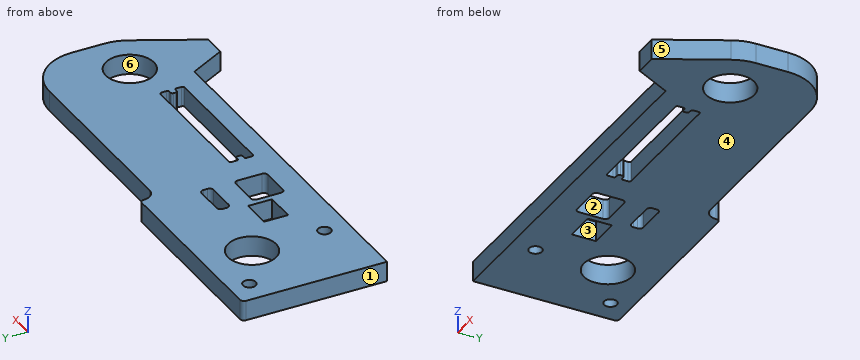
```python
from build123d import *

# Parameters (mm, degrees)
SKETCH1_R           = 5.98
SKETCH1_R_2         = 1.6
SKETCH1_W           = 9
SKETCH1_H           = 8
SKETCH1_H_2         = 3
SKETCH1_W_2         = 7.5
SKETCH1_H_3         = 6
BOSS_EXTRUDE1_DEPTH = 5
FILLET1_R           = 1
FILLET2_R           = 3
FILLET3_R           = 1
CUT_EXTRUDE1_DEPTH  = 98.867257037
FILLET4_R           = 0.5


with BuildPart() as part:
    # Sketch1 → Boss-Extrude1 (new body)
    with BuildSketch(Plane.XY):
        with BuildLine():
            Line((72.356568311, -24), (77.172081726, -33))
            Line((77.172081726, -33), (82.827918274, -33))
            Line((82.827918274, -33), (90.70873293, -17.415075165))
            ThreePointArc((90.70873293, -17.415075165), (91.67272023, -14.78345153), (92, -12))
            Line((92, -12), (92, -4))
            ThreePointArc((92, -4), (88.485281374, 4.485281374), (80, 8))
            Line((80, 8), (30, 8))
            Line((30, 8), (30, 12))
            Line((30, 12), (-18, 12))
            Line((-18, 12), (-18, -24))
            Line((-18, -24), (72.356568311, -24))
        make_face()
        Circle(SKETCH1_R, mode=Mode.SUBTRACT)
        with Locations((80, -12)):
            Circle(SKETCH1_R, mode=Mode.SUBTRACT)
        with Locations((-12, 7)):
            Circle(SKETCH1_R_2, mode=Mode.SUBTRACT)
        with Locations((0, -18)):
            Circle(SKETCH1_R_2, mode=Mode.SUBTRACT)
        with Locations((23, -14)):
            Rectangle(SKETCH1_W, SKETCH1_H, mode=Mode.SUBTRACT)
        with Locations((23, -3)):
            Rectangle(SKETCH1_W, SKETCH1_H_2, mode=Mode.SUBTRACT)
        with Locations((13.25, -11)):
            Rectangle(SKETCH1_W_2, SKETCH1_H_3, mode=Mode.SUBTRACT)
    extrude(amount=BOSS_EXTRUDE1_DEPTH)

    # Fillet1
    fillet1_edges = [part.edges().sort_by_distance(p)[0] for p in [
        (18.5, -10, 2.5),
        (18.5, -18, 2.5),
        (27.5, -18, 2.5),
        (27.5, -10, 2.5),
        (18.5, -1.5, 2.5),
        (18.5, -4.5, 2.5),
        (27.5, -4.5, 2.5),
        (27.5, -1.5, 2.5),
    ]]
    fillet(fillet1_edges, radius=FILLET1_R)

    # Fillet2
    fillet2_edges = [part.edges().sort_by_distance(p)[0] for p in [
        (30, 8, 2.5),
    ]]
    fillet(fillet2_edges, radius=FILLET2_R)

    # Fillet3
    fillet3_edges = [part.edges().sort_by_distance(p)[0] for p in [
        (30, 12, 2.5),
        (-18, 12, 2.5),
    ]]
    fillet(fillet3_edges, radius=FILLET3_R - 0.0001)  # a hair under: the kernel refuses the full size

    # Sketch2 → Cut-Extrude1 (cut, through all)
    with BuildSketch(Plane.XY.offset(5)):
        Polygon((35, -13), (68, -13), (68, -15.25), (66.5, -15.25), (66.5, -16.75), (68, -16.75), (68, -19), (35, -19), (35, -16.75), (36.5, -16.75), (36.5, -15.25), (35, -15.25), align=None)
    extrude(amount=-CUT_EXTRUDE1_DEPTH, mode=Mode.SUBTRACT)

    # Fillet4
    fillet4_edges = [part.edges().sort_by_distance(p)[0] for p in [
        (35, -15.25, 2.5),
        (35, -13, 2.5),
        (68, -13, 2.5),
        (68, -15.25, 2.5),
        (66.5, -15.25, 2.5),
        (66.5, -16.75, 2.5),
        (68, -16.75, 2.5),
        (68, -19, 2.5),
        (35, -19, 2.5),
        (35, -16.75, 2.5),
        (36.5, -16.75, 2.5),
        (36.5, -15.25, 2.5),
    ]]
    fillet(fillet4_edges, radius=FILLET4_R)


solid = part.part
```
Input: part model. Units: mm. Frame: model coordinates. Face numbers are marked on the shaded views. A direction names the side the tool comes from. Coordinates: 2 decimals unless noted, no trailing zeros. Loops run counter-clockwise (first coordinate to the right, second up) from the corner with the lowest first, then second, coordinate; pieces in that order, holes last. Notation, with made-up numbers: M 11,60.5 L 23,60.5 A31 cw 23,84.5 Z; hole C 52,-32 d10. An arc over 180 degrees is marked long. Answer in a Markdown table with one row per item.
1. Section A-A, the plane x = 46. Output: boundary loops of the cut face in (y, z).
Response:
| item | result |
|---|---|
| outline | M -24,0 L -19,0 L -19,5 L -24,5 Z; M -13,0 L 8,0 L 8,5 L -13,5 Z |
2. First-contact query: pin 1 (2 mm diameter, centred on x = 27, y = 3, fed in from -Z); pin 2 (11 mm diameter, centred on x = 0, y = 0, fed in from +Z); pin 3 (1 mm diameter, centred on x = 32, z = 2, fed in from -Y); pin 4 (0.6 mm diameter, centred on y = -18, z = 3, fed in from +X). Flat tips, straight axial feed; report the tip coordinate or a pass-through.
Response:
| item | result |
|---|---|
| pin 1 | stops at z = 0 |
| pin 2 | passes through |
| pin 3 | stops at y = -24 |
| pin 4 | stops at x = 90.56 |
3. Section D-D, the plane z = 2.6. Count the separate pieces of the cut face and the enclosed holes in it, then the cut area to 3 significant figures.
Response:
| item | result |
|---|---|
| separate pieces | 1 |
| enclosed holes | 8 |
| area | 3,180 mm2 |
4. Section B-B, the plane x = 0. Output: boundary loops of the cut face in (y, z), then the cut area to 3 significant figures.
Response:
| item | result |
|---|---|
| outline | M -24,0 L -19.6,0 L -19.6,5 L -24,5 Z; M -16.4,0 L -5.98,0 L -5.98,5 L -16.4,5 Z; M 5.98,0 L 12,0 L 12,5 L 5.98,5 Z |
| area | 104 mm2 |
5. Section C-C, the plane y = 0. Output: boundary loops of the cut face in (x, z), then the cut area to 3 significant figures.
Response:
| item | result |
|---|---|
| outline | M -18,0 L -5.98,0 L -5.98,5 L -18,5 Z; M 5.98,0 L 91.31,0 L 91.31,5 L 5.98,5 Z |
| area | 487 mm2 |
6. Draft query along Y for the marked faces 3, 4, 5 and 6. Return one class per face: pulls with the +Y half, pulls with the -Y half, needs draft (parallel to the pull), parting line crosses it, or undercut.
Response:
| item | result |
|---|---|
| face 3 | undercut |
| face 4 | needs draft |
| face 5 | pulls with the -Y half |
| face 6 | undercut |
7. Reachability of the marked faces 1 and 2 from +Z, -Z, +X, -X, +Y, -Y: full face, straight path, thin tool, end or side. Return the list, or none.
Response:
| item | result |
|---|---|
| face 1 | +Z, -Z, -X, +Y, -Y |
| face 2 | +Z, -Z |
8. Material intervals for line 1 (Y direction, x = 0, z = 3.2); line 2 (Y direction, x = 80, z = 3.5); line 3 (Y direction, x = 59.5, z = 1.8), sorted ascending.
Response:
| item | result |
|---|---|
| line 1 | y = -24 to -19.6, -16.4 to -5.98, 5.98 to 12 |
| line 2 | y = -33 to -17.98, -6.02 to 8 |
| line 3 | y = -24 to -19, -13 to 8 |
